Could you check a few things on this drawing? It's one solid part, dimensions in mm from its lowest x, y, z. Give positions to 0.01 mm unless a question says otherwise; leave off trailing zeros. Order: outer loops, then holes, each group sorted by start corner. A loop starts at its lowest first (then second) coordinate and runs counter-clockwise, first axis right, second up. Notation, with made-up numbers: M -0.5,-32 L 42.5,-32 A13 ccw 42.5,-25 Z; hole C 7.5,4.5 d10. An arc over 180 degrees is marked long. Use one line per item in the form item = value.
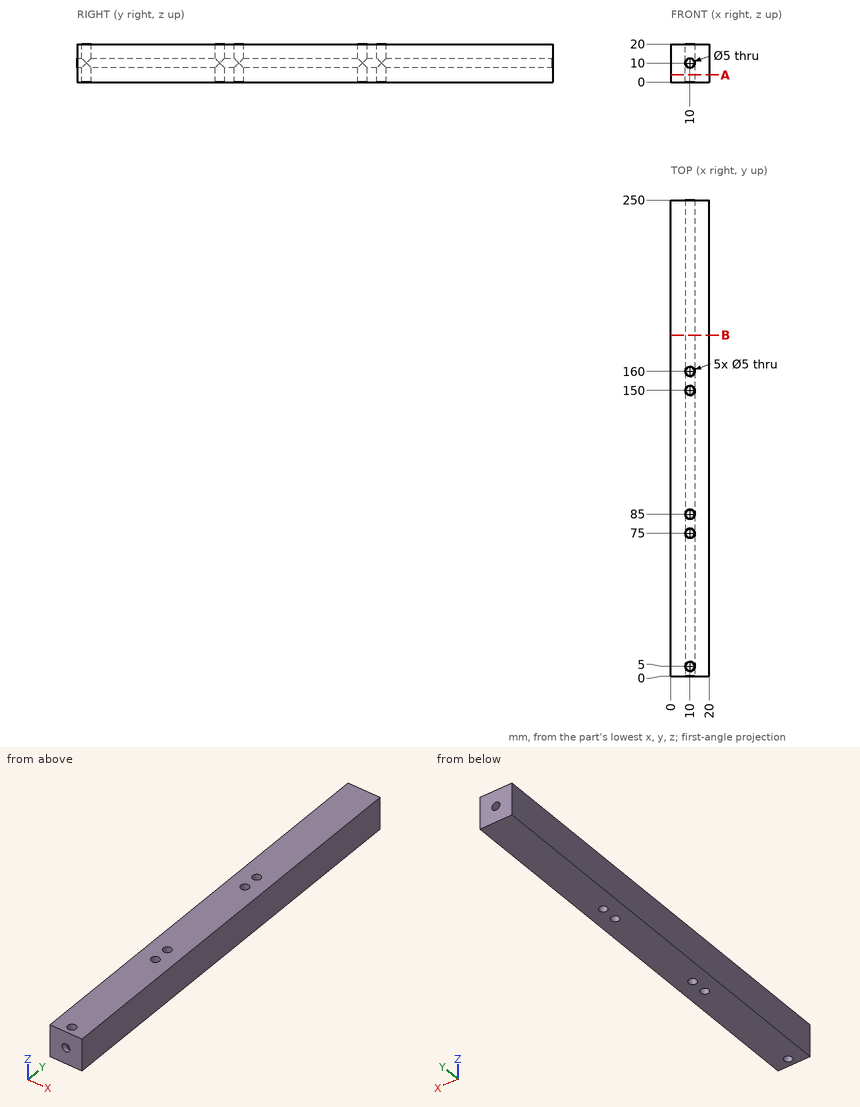
Q1. I want a section at B-B on y = 179. Write out the boundary of the cut face in (x, z), then the cut area to 3 significant figures.
Found:
outline = M 0,0 L 20,0 L 20,20 L 0,20 Z; hole C 10,10 d5
area = 380 mm²
Q2. I want a section at A-A on z = 3.75. Write out the boundary of the cut face in (x, y), then the cut area to 3 significant figures.
Found:
outline = M 0,0 L 20,0 L 20,250 L 0,250 Z; hole C 10,5 d5; hole C 10,75 d5; hole C 10,85 d5; hole C 10,150 d5; hole C 10,160 d5
area = 4,900 mm²
Q3. I need wall thicknesses on L1, parallel to Y at x = 10, z = 2.25; L2, parallel to X at y = 85, z = 3.5; L3, parallel to Y at x = 10.75, z = 5.25. Which ranges of each line are inside material? Lowest first, please.
Found:
L1 = 0 to 2.5, 7.5 to 72.5, 77.5 to 82.5, 87.5 to 147.5, 152.5 to 157.5, 162.5 to 250
L2 = 0 to 7.5, 12.5 to 20
L3 = 0 to 2.62, 7.38 to 72.62, 77.38 to 82.62, 87.38 to 147.62, 152.38 to 157.62, 162.38 to 250
